Read the model definition and answer for the solid it produces. Units are mm, in the model's axes. Face numbers are marked on the shaded views. Coordinates: 2 decimals unless noted, no trailing zeros. Loops run counter-clockwise (first coordinate to the right, second up) from the corner with the lowest first, then second, coordinate; pieces in that order, holes last. Notation, with made-up numbers: (-3, -29.5) -> (27, -29.5) arc R23 ccw to (27, -13.5) -> close; hole circle Ø6 at (-15, 57). An arc over 180 degrees is marked (long way). Answer in a Markdown table with one row per item.
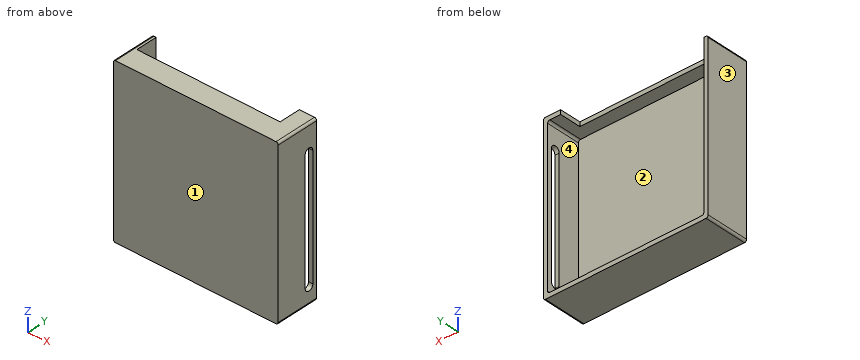
```python
from build123d import *

# Parameters (mm, degrees)
BOSS_EXTRUDE2_DEPTH = 50
BOSS_EXTRUDE3_DEPTH = 10
CUT_EXTRUDE1_DEPTH  = 10
SKETCH4_W           = 140
SKETCH4_H           = 10
CUT_EXTRUDE2_DEPTH  = 10


with BuildPart() as part:
    # Sketch1 → Boss-Extrude2 (new body)
    with BuildSketch(Plane(origin=(0, 0, 0), x_dir=(1, 0, 0), z_dir=(0, 1, 0))):
        with BuildLine():
            Line((-93, 95.5), (93, 95.5))
            ThreePointArc((93, 95.5), (94.767766953, 94.767766953), (95.5, 93))
            Line((95.5, 93), (95.5, -93))
            ThreePointArc((95.5, -93), (94.767766953, -94.767766953), (93, -95.5))
            Line((93, -95.5), (-93, -95.5))
            ThreePointArc((-93, -95.5), (-94.767766953, -94.767766953), (-95.5, -93))
            Line((-95.5, -93), (-95.5, 93))
            ThreePointArc((-95.5, 93), (-94.767766953, 94.767766953), (-93, 95.5))
        make_face()
        with BuildLine():
            Line((-88, 90.5), (88, 90.5))
            ThreePointArc((88, 90.5), (89.767766953, 89.767766953), (90.5, 88))
            Line((90.5, 88), (90.5, -88))
            ThreePointArc((90.5, -88), (89.767766953, -89.767766953), (88, -90.5))
            Line((88, -90.5), (-88, -90.5))
            ThreePointArc((-88, -90.5), (-89.767766953, -89.767766953), (-90.5, -88))
            Line((-90.5, -88), (-90.5, 88))
            ThreePointArc((-90.5, 88), (-89.767766953, 89.767766953), (-88, 90.5))
        make_face(mode=Mode.SUBTRACT)
    extrude(amount=BOSS_EXTRUDE2_DEPTH)

    # Sketch2 → Boss-Extrude3 (add)
    with BuildSketch(Plane(origin=(0, 0, 0), x_dir=(1, 0, 0), z_dir=(0, 1, 0))):
        with BuildLine():
            Line((-88, 90.5), (88, 90.5))
            ThreePointArc((88, 90.5), (89.767766953, 89.767766953), (90.5, 88))
            Line((90.5, 88), (90.5, -88))
            ThreePointArc((90.5, -88), (89.767766953, -89.767766953), (88, -90.5))
            Line((88, -90.5), (-88, -90.5))
            ThreePointArc((-88, -90.5), (-89.767766953, -89.767766953), (-90.5, -88))
            Line((-90.5, -88), (-90.5, 88))
            ThreePointArc((-90.5, 88), (-89.767766953, 89.767766953), (-88, 90.5))
        make_face()
    extrude(amount=BOSS_EXTRUDE3_DEPTH)

    # Sketch3 → Cut-Extrude1 (cut)
    with BuildSketch(Plane.XY.offset(95.5)):
        Polygon((-90.5, 25), (0, 25), (75.5, 25), (75.5, 50), (-90.5, 50), align=None)
    extrude(amount=-CUT_EXTRUDE1_DEPTH, mode=Mode.SUBTRACT)

    # Sketch4 → Cut-Extrude2 (cut)
    with BuildSketch(Plane(origin=(95.5, 0, 0), x_dir=(0, 0, -1), z_dir=(1, 0, 0))):
        with Locations((5.5, 40)):
            Rectangle(SKETCH4_W, SKETCH4_H)
        with BuildLine():
            Line((75.5, 35), (75.5, 45))
            ThreePointArc((75.5, 45), (80.5, 40), (75.5, 35))
        make_face()
        with BuildLine():
            Line((-64.5, 35), (-64.5, 45))
            ThreePointArc((-64.5, 45), (-69.5, 40), (-64.5, 35))
        make_face()
    extrude(amount=-CUT_EXTRUDE2_DEPTH, mode=Mode.SUBTRACT)


solid = part.part
```
1. A cutting plane is placed at C-C on x = 41. Give the vertices of the cut face in (y, z), and give its area (4 significant figures).
A:
| item | result |
|---|---|
| outline | (0, -95.5) -> (50, -95.5) -> (50, -90.5) -> (10, -90.5) -> (10, 90.5) -> (25, 90.5) -> (25, 95.5) -> (0, 95.5) -> close |
| area | 2,185 mm2 |
2. A cutting plane is placed at B-B on y = 40. Give the vertices of the cut face in (x, z).
A:
| item | result |
|---|---|
| outline | (-95.5, -93) arc R2.5 ccw to (-93, -95.5) -> (93, -95.5) arc R2.5 ccw to (95.5, -93) -> (95.5, -80.5) -> (90.5, -80.5) -> (90.5, -88) arc R2.5 cw to (88, -90.5) -> (-88, -90.5) arc R2.5 cw to (-90.5, -88) -> (-90.5, 95.5) -> (-93, 95.5) arc R2.5 ccw to (-95.5, 93) -> close; (75.5, 90.5) -> (88, 90.5) arc R2.5 cw to (90.5, 88) -> (90.5, 69.5) -> (95.5, 69.5) -> (95.5, 93) arc R2.5 ccw to (93, 95.5) -> (75.5, 95.5) -> close |
3. The mould has two halves that part along X. Classify the marked faces 1, 2, 3 and 4: pulls with the +X half, pulls with the -X half, needs draft (parallel to the pull), parting line crosses it, or undercut.
A:
| item | result |
|---|---|
| face 1 | needs draft |
| face 2 | undercut |
| face 3 | pulls with the -X half |
| face 4 | undercut |
4. A cutting plane is placed at A-A on z = 11.5. Give the vertices of the cut face in (x, y).
A:
| item | result |
|---|---|
| outline | (-95.5, 0) -> (95.5, 0) -> (95.5, 35) -> (90.5, 35) -> (90.5, 10) -> (-90.5, 10) -> (-90.5, 50) -> (-95.5, 50) -> close; (90.5, 45) -> (95.5, 45) -> (95.5, 50) -> (90.5, 50) -> close |
5. Find the intervals of material crossed by probe 1 along X at (y, z) = (20.5, -71.5); probe 2 along Y at (x, z) = (-80.5, 79), in increasing order.
A:
| item | result |
|---|---|
| probe 1 | x = -95.5 to -90.5, 90.5 to 95.5 |
| probe 2 | y = 0 to 10 |
6. A cutting plane is placed at D-D on y = 15.5. Give the vertices of the cut face in (x, z).
A:
| item | result |
|---|---|
| outline | (-95.5, -93) arc R2.5 ccw to (-93, -95.5) -> (93, -95.5) arc R2.5 ccw to (95.5, -93) -> (95.5, 93) arc R2.5 ccw to (93, 95.5) -> (-93, 95.5) arc R2.5 ccw to (-95.5, 93) -> close; hole (-90.5, -88) arc R2.5 ccw to (-88, -90.5) -> (88, -90.5) arc R2.5 ccw to (90.5, -88) -> (90.5, 88) arc R2.5 ccw to (88, 90.5) -> (-88, 90.5) arc R2.5 ccw to (-90.5, 88) -> close |
7. Given pin 1 Ø10 at (x, z) = (-65.5, -1.5) entering from +Y; pin 2 Ø6 at (x, z) = (-3.5, 93) entering from +Y, each flat-ended and moving along its own axis, determine where each tip first touches the part or whether it passes through.
A:
| item | result |
|---|---|
| pin 1 | stops at y = 10 |
| pin 2 | stops at y = 25 |
